Could you check a few things on this drawing? It's one solid part, dimensions in mm from its lowest x, y, z. A direction names the side the tool comes from. Give positions to 0.01 mm unless a question says otherwise; leave off trailing zeros. Loops run counter-clockwise (first coordinate to the right, second up) from the corner with the lowest first, then second, coordinate; pieces in that order, holes last. Notation, with made-up numbers: M 59.5,33 L 111.5,33 A33 cw 111.5,69 Z; hole C 82,-34.5 d3. An arc over 180 degrees is marked long. Answer in a Markdown table with one row per item. Add a question column.
1. If we section it at B-B on z = 57: List the corners of the cut face in (x, y) for me.
2. Which directions (+Z, -Z, +X, -X, +Y, -Y) give clear straight access to the entire face, cutting with the end or side of a thin tool? Please do the marked faces 1 and 2.
3. If we section it at A-A on z = 26.5: List the corners of the cut face in (x, y) for me, then the cut area to 3 significant figures.
4. I'm going to push flat-ended pins straight in: pin 1 Ø4 at (y, z) = (8, 16) entering from -X; pin 2 Ø1.5 at (x, y) = (9, 4.5) entering from -Z; pin 3 Ø5 at (y, z) = (5.5, 28) entering from +X. Where does each tip first touch, or does it pass through?
5. I need wall thicknesses on line 1 along Z through (x, y) = (8, 2.5); line 2 along Y through (x, z) = (1, 75); line 3 along X through (y, z) = (4.75, 48). Which ranges of each line are inside material? Lowest first, please. Write a range as from..to.
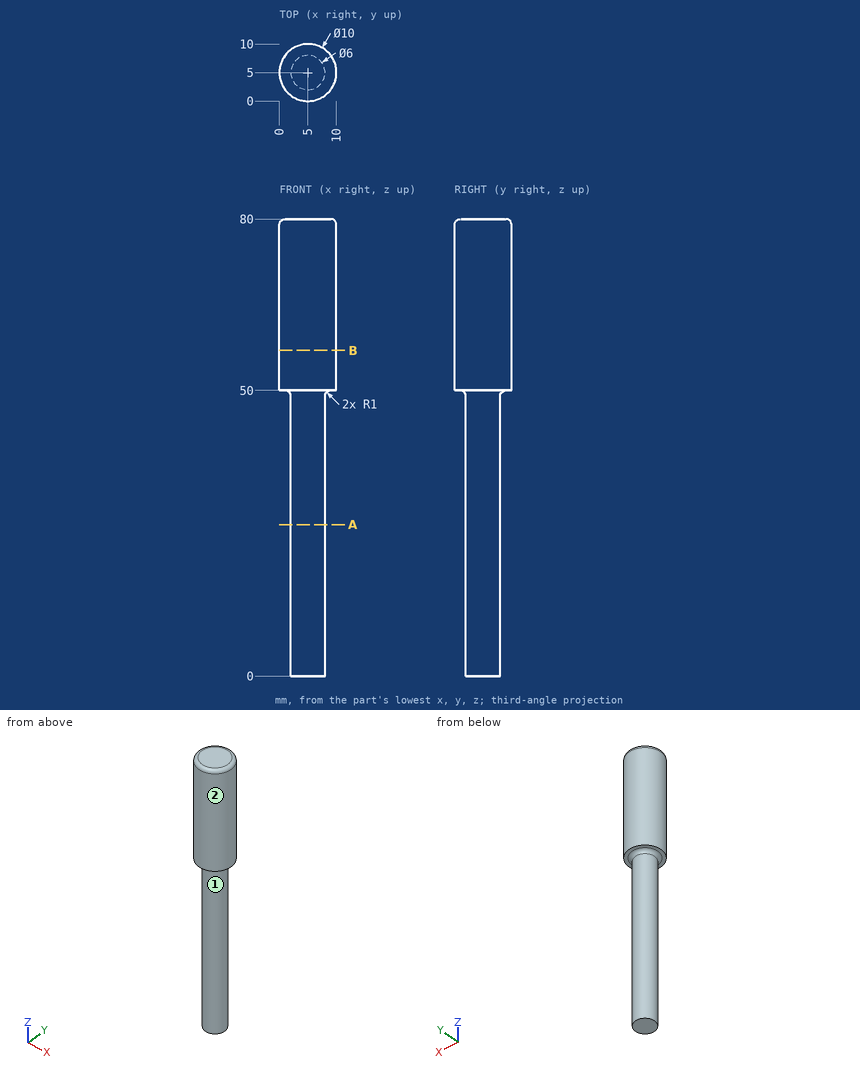
Results:
| question | item | result |
|---|---|---|
| 1 | outline | C 5,5 d10 |
| 2 | face 1 | -Z |
| 2 | face 2 | +Z, -Z |
| 3 | outline | C 5,5 d6 |
| 3 | area | 28.3 mm2 |
| 4 | pin 1 | x = 2.17 |
| 4 | pin 2 | z = 49.7 |
| 4 | pin 3 | x = 8 |
| 5 | line 1 | 50..80 |
| 5 | line 2 | 2..8 |
| 5 | line 3 | 2.01..7.99 |
